Could you check a few things on this model? Use its own coordinates, in mm. A direction names the side the tool comes from. Round coordinates to 2 decimals unless told otherwise and drop trailing zeros. Loops run counter-clockwise (first coordinate to the right, second up) from the corner with the lowest first, then second, coordinate; pieces in that order, holes last. Notation, with made-up numbers: M 49.25,26.25 L 69.25,26.25 A19 ccw 69.25,37.25 Z; hole C -39.5,11 d2. An arc over 180 degrees is marked long. Return JSON: item names as keys, results as strings. Group by question number.
```python
from build123d import *

# Parameters (mm, degrees)
BOSS_EXTRUDE1_DEPTH = 10
FILLET1_R           = 4.572


with BuildPart() as part:
    # Sketch2 → Boss-Extrude1 (new body)
    with BuildSketch(Plane(origin=(0, 0, 0), x_dir=(1, 0, 0), z_dir=(0, 1, 0))):
        with BuildLine():
            Line((6.098836138, 199.947644416), (7.673025909, 77.750683868))
            Line((7.673025909, 77.750683868), (24.192411242, 61.855234605))
            Line((24.192411242, 61.855234605), (24.192411242, 48.766267951))
            Line((24.192411242, 48.766267951), (1.672918099, 48.766267951))
            Line((1.672918099, 48.766267951), (1.672918099, 36.564568547))
            Line((1.672918099, 36.564568547), (36.816624548, 36.564568547))
            Line((36.816624548, 36.564568547), (36.816624548, 61.855234605))
            Line((36.816624548, 61.855234605), (50.677233754, 77.750683868))
            Line((50.677233754, 77.750683868), (51.925307167, 200.008903269))
            ThreePointArc((51.925307167, 200.008903269), (28.981086555, 223.157579607), (6.098836138, 199.947644416))
        make_face()
    extrude(amount=BOSS_EXTRUDE1_DEPTH)

    # Fillet1
    fillet1_edges = [part.edges().sort_by_distance(p)[0] for p in [
        (36.816624548, 0, -49.209901576),
        (19.244771323, 0, -36.564568547),
        (12.932664671, 0, -48.766267951),
        (24.192411242, 0, -55.310751278),
        (24.192411242, 10, -55.310751278),
        (12.932664671, 10, -48.766267951),
        (19.244771323, 10, -36.564568547),
        (36.816624548, 10, -49.209901576),
    ]]
    fillet(fillet1_edges, radius=FILLET1_R)


solid = part.part
```
1. On a 3-axis mill with a long thin cutter (end or side, diameter ignored), from which of +Z, -Z, +X, -X, +Y, -Y can I reach the whole of each face in a straight line? I mean faces 4 (the face through (35.51, 1.37, -49.39)), 5 (the face through (15.03, 8.63, -47.46)), 6 (the face through (25.5, 1.37, -52.9)). Say none if no direction works.
2. If we section it at D-D, the plane x = 20.5: Please give me the cut outline in (y, z).
3. If we section it at A-A, the plane x = 12.5: Please give me the cut outline in (y, z), then the cut area to 3 significant figures.
4. I need wall thicknesses on probe 1 along Z at (x, y) = (5, 5); probe 2 along Z at (x, y) = (30, 4); probe 3 along Z at (x, y) = (21, 4). Which ranges of each line are inside material? Lowest first, please.
5. I'm going to push flat-ended pins straight in: pin 1 Ø1.5 at (y, z) = (1.5, -94) entering from +X; pin 2 Ø3 at (y, z) = (4, -178.5) entering from +X; pin 3 Ø6 at (y, z) = (4, -174) entering from -X. Where does each tip first touch, or does it pass through?
6. We'd pull the mould along Z, two halves only. Please class faces 1 (the face through (32, 10, -133)), 2 (the face through (19.491, 1.375, -37.868)), 3 (the face through (15.73, 4.93, -70)): +Z half, -Z half, draft (parallel to the pull), parting line (faces both ways), or undercut.
7. If we section it at C-C, the plane y = 8: Please give me the cut outline in (x, z).
8. If we section it at B-B, the plane z = -55: Please give me the cut outline in (x, y).
Geometry results:
{
 "1": {"face 4": "+Z, +X, -Y", "face 5": "-X, +Y", "face 6": "-X, -Y"},
 "2": {"outline": "M 0,-221.52 L 10,-221.52 L 10,-65.41 L 0,-65.41 Z; M 0,-44.19 A4.57 ccw 4.57,-48.77 L 5.43,-48.77 A4.57 ccw 10,-44.19 L 10,-41.14 A4.57 ccw 5.43,-36.56 L 4.57,-36.56 A4.57 ccw 0,-41.14 Z"},
 "3": {"outline": "M 0,-216.13 L 10,-216.13 L 10,-73.11 L 0,-73.11 Z; M 0,-44.19 A4.57 ccw 4.57,-48.77 L 5.43,-48.77 A4.57 ccw 10,-44.19 L 10,-41.14 A4.57 ccw 5.43,-36.56 L 4.57,-36.56 A4.57 ccw 0,-41.14 Z", "area": "1,530 mm^2"},
 "4": {"probe 1": "-48.77 to -36.56", "probe 2": "-223.14 to -36.6", "probe 3": "-221.71 to -64.93, -48.73 to -36.6"},
 "5": {"pin 1": "x = 50.85", "pin 2": "x = 51.72", "pin 3": "x = 6.39"},
 "6": {"face 1": "draft", "face 2": "+Z half", "face 3": "undercut"},
 "7": {"outline": "M 1.67,-47.97 L 24.98,-47.97 L 24.98,-61.09 L 7.67,-77.75 L 6.1,-199.95 A22.91 ccw long 51.93,-200.01 L 50.68,-77.75 L 36.02,-60.95 L 36.02,-37.36 L 1.67,-37.36 Z"},
 "8": {"outline": "M 24.19,4.57 A4.57 ccw 28.76,0 L 32.24,0 A4.57 ccw 36.82,4.57 L 36.82,5.43 A4.57 ccw 32.24,10 L 28.76,10 A4.57 ccw 24.19,5.43 Z"}
}
